Source: three-view drawing plus pictorial views. Frame: mm from the lowest corner of the part. Coordinates: 2 decimals unless noted, no trailing zeros. Write each loop counter-clockwise with the first axis right and the second up, starting at its lowest first coordinate (ties: lowest second). Pieces come first, ordered by that corner, then holes. Notation, with made-up numbers: M 60.5,54.5 L 77.5,54.5 A22 cw 77.5,90.5 Z; hole C 34.5,86 d8. An arc over 180 degrees is marked long. Write item = value, one per line. Start each with the question number.
Item 1: Pull-direction query (X, two-part tool) for the marked faces 1, 2 and 3; classes: +X half, -X half, draft (parallel to the pull), parting line (faces both ways), or undercut.
Item 2: Section D-D on x = 7. Output: boundary loops of the cut face in (y, z).
Item 3: Section B-B on x = 25.4. Output: boundary loops of the cut face in (y, z) (1 decimal).
Item 4: Ray query, L1, parallel to Y at x = 20.5, z = 43.5; L2, parallel to Z at x = 26, y = 7.25 (1 decimal); L3, parallel to Z at x = 29, y = 1.25 (1 decimal). Return the intervals inside material, ascending. Write a range as [from, to].
Item 5: First-contact query: pin 1 Ø4 at (x, y) = (40, 6.5) entering from +Z (1 decimal); pin 2 Ø3 at (y, z) = (12, 27.5) entering from +X; pin 3 Ø5 at (x, y) = (21.5, 16) entering from +Z. Flat tips, straight axial feed; report the tip coordinate or a pass-through.
Item 6: Section C-C on y = 20.5. Output: boundary loops of the cut face in (x, z) (1 decimal).
Item 7: Section A-A on z = 25.4. Output: boundary loops of the cut face in (x, y) (1 decimal).
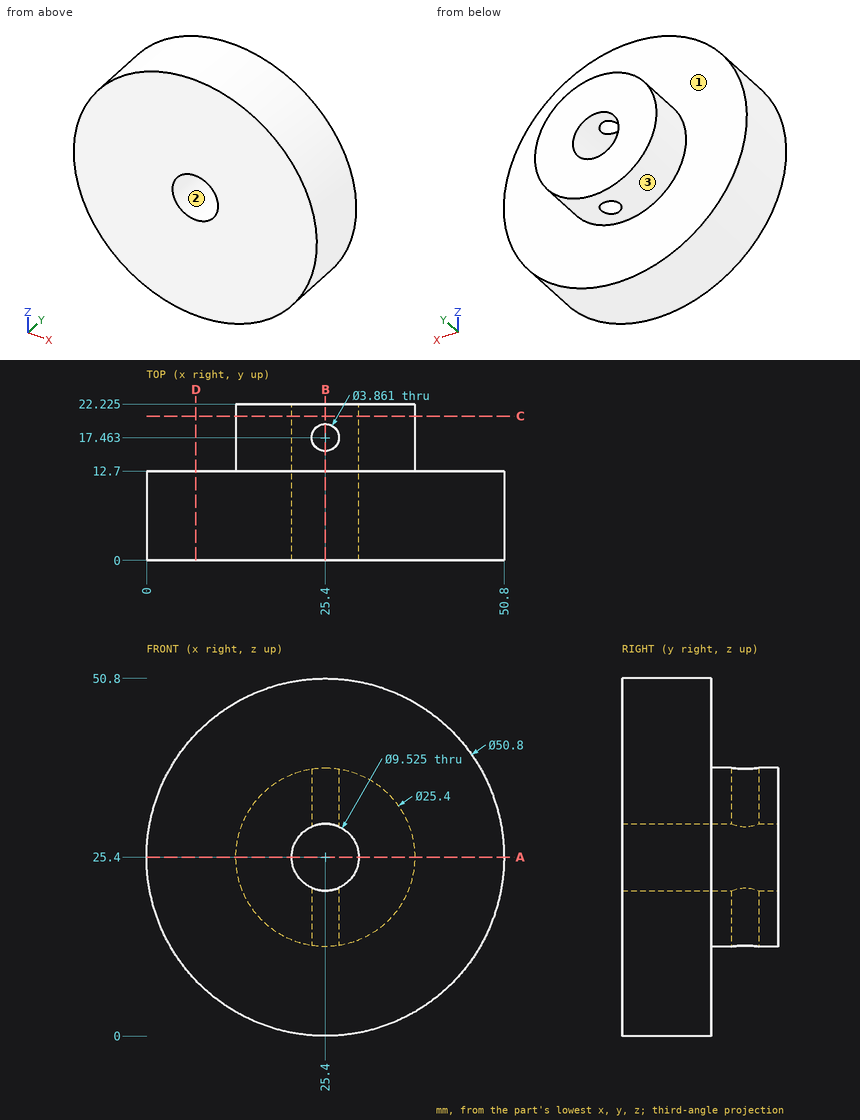
Responses:
q1.face_1 = draft
q1.face_2 = undercut
q1.face_3 = parting line
q2.outline = M 0,7.89 L 12.7,7.89 L 12.7,42.91 L 0,42.91 Z
q3.outline = M 0,0 L 12.7,0 L 12.7,12.7 L 15.5,12.7 L 15.5,20.6 L 0,20.6 Z; M 0,30.2 L 15.5,30.2 L 15.5,38.1 L 12.7,38.1 L 12.7,50.8 L 0,50.8 Z; M 19.4,12.7 L 22.2,12.7 L 22.2,20.6 L 19.4,20.6 Z; M 19.4,30.2 L 22.2,30.2 L 22.2,38.1 L 19.4,38.1 Z
q4.L1 = [0, 12.7]
q4.L2 = [0, 20.7], [30.1, 50.8]
q4.L3 = [0.3, 22.3], [28.5, 50.5]
q5.pin_1 = 47.5
q5.pin_2 = 50.79
q5.pin_3 = 38.02
q6.outline = C 25.4,25.4 d25.4; hole C 25.4,25.4 d9.5
q7.outline = M 0,0 L 20.6,0 L 20.6,22.2 L 12.7,22.2 L 12.7,12.7 L 0,12.7 Z; M 30.2,0 L 50.8,0 L 50.8,12.7 L 38.1,12.7 L 38.1,22.2 L 30.2,22.2 Z
